The model under review builds one solid part; all positions refer to its coordinate system, in mm. A direction names the side the tool comes from. Coordinates: 2 decimals unless noted, no trailing zeros. Order: outer loops, then holes, each group sorted by start corner. A loop starts at its lowest first (then second) coordinate and runs counter-clockwise, first axis right, second up. Notation, with made-up numbers: (-5, 1) -> (49, 1) arc R20 ccw to (49, 35) -> close; hole circle Ø8 at (-9.75, 29.25). An arc over 180 degrees is marked (long way). Use one line per item in the form item = value. Start each with the question number.
(1) Wall thickness on line 1 along X through (y, z) = (22.5, 10); line 2 along X through (y, z) = (29, 23.75); line 3 along Y through (x, z) = (14, 2.5): over which ranges is each line inside the solid? List them lowest first.
(2) Take a section at C-C (x = 1). State the section outline as (y, z) points.
(3) Take a section at A-A (z = 22.5). State the section outline as (x, y) points, then the cut area to 3 significant figures.
(4) For faces 1 (the cylindrical face through (14.79, 14.894, 22.42)), 2 (the cylindrical face through (-27.32, 22.52, 12.83)), 3 (the flat face through (-8, 0, 12)), 4 (the flat face through (0, 32, 3)), 5 (the flat face through (0, 32, 22)), list the 3-axis set-ups (+Z, -Z, +X, -X, +Y, -Y) from which the entire face can be reached by the end or side of a thin tool; tool diameter is ignored.
(5) Take a section at D-D (y = 4). State the section outline as (x, z) points.
(6) Take a section at B-B (y = 12.5). State the section outline as (x, z) points, then the cut area to 3 significant figures.
(7) Insertion check: pin 1 Ø11 at (y, z) = (6, 7.5) entering from +X; pin 2 Ø6 at (x, z) = (22, 4.5) entering from -Y; pin 3 Ø6 at (x, z) = (15.5, 8) entering from -Y; pin 4 Ø4 at (x, z) = (-23, 6.5) entering from -Y. Each pin has a flat end and moves straight along its axis. Give the tip position at first contact, or say it passes through.
```python
from build123d import *

# Parameters (mm, degrees)
ESQUISSE1_W             = 15
ESQUISSE1_H             = 35
EXTRUSION1_DEPTH        = 25
ESQUISSE2_R             = 12.5
EXTRUSION2_DEPTH        = 30
ESQUISSE3_R             = 2.5
EXTRUSION4_DEPTH        = 25
ESQUISSE4_W             = 5.704163369
ESQUISSE4_H             = 5
ENL_V_MAT_EXTRU_1_DEPTH = 0.0001
ESQUISSE5_W             = 5.704163369
ESQUISSE5_H             = 5
ENL_V_MAT_EXTRU_2_DEPTH = 0.0001


with BuildPart() as part:
    # Esquisse1 → Extrusion1 (new body)
    with BuildSketch(Plane.XY):
        with Locations((-7.5, 17.5)):
            Rectangle(ESQUISSE1_W, ESQUISSE1_H)
    extrude(amount=EXTRUSION1_DEPTH)

    # Esquisse2 → Extrusion2 (add)
    with BuildSketch(Plane(origin=(0, 0, 0), x_dir=(0, 0, -1), z_dir=(1, 0, 0))):
        with Locations((-12.5, 22.5)):
            Circle(ESQUISSE2_R)
    extrude(amount=EXTRUSION2_DEPTH)

    # Esquisse3 → Extrusion4 (add)
    with BuildSketch(Plane.ZY.offset(15)):
        with Locations(Location((12.5, 25, 0), (0, 0, 180))):
            Circle(ESQUISSE3_R)
    extrude(amount=EXTRUSION4_DEPTH)

    # Esquisse4 → Enlèv. mat.-Extru.1 (cut)
    with BuildSketch(Plane.XY.offset(25)):
        with Locations((-12.147918316, 25)):
            Rectangle(ESQUISSE4_W, ESQUISSE4_H)
    extrude(amount=-ENL_V_MAT_EXTRU_1_DEPTH, mode=Mode.SUBTRACT)

    # Esquisse5 → Enlèv. mat.-Extru.2 (cut)
    with BuildSketch(Plane(origin=(0, 0, 0), x_dir=(-1, 0, 0), z_dir=(0, 0, -1))):
        with Locations((12.129729433, 24.948694164)):
            Rectangle(ESQUISSE5_W, ESQUISSE5_H)
    extrude(amount=-ENL_V_MAT_EXTRU_2_DEPTH, mode=Mode.SUBTRACT)


solid = part.part
```
Findings:
q1.line_1 = -15 to 30
q1.line_2 = -15 to 0
q1.line_3 = 15 to 30
q2.outline = circle Ø25 at (22.5, 12.5)
q3.outline = (-15, 0) -> (0, 0) -> (0, 15) -> (30, 15) -> (30, 30) -> (0, 30) -> (0, 35) -> (-15, 35) -> close
q3.area = 975 mm²
q4.face_1 = +X
q4.face_2 = -X
q4.face_3 = +Z, -Z, +X, -X, -Y
q4.face_4 = -Z, +X, +Y
q4.face_5 = +Z, +X, +Y
q5.outline = (-15, 0) -> (0, 0) -> (0, 25) -> (-15, 25) -> close
q6.outline = (-15, 0) -> (0, 0) -> (0, 5) -> (30, 5) -> (30, 20) -> (0, 20) -> (0, 25) -> (-15, 25) -> close
q6.area = 825 mm²
q7.pin_1 = 30
q7.pin_2 = 11.04
q7.pin_3 = 10.09
q7.pin_4 = through
